Here's how the part is built. I have some questions about the finished solid (model axes, mm). Face numbers are marked on the shaded views. A direction names the side the tool comes from. Round coordinates to 2 decimals unless told otherwise and drop trailing zeros. Order: outer loops, then holes, each group sorted by start corner. A loop starts at its lowest first (then second) coordinate and runs counter-clockwise, first axis right, second up. Notation, with made-up numbers: M 30,69 L 82,69 A21 ccw 82,102 Z; hole C 1.5,19 d10. An arc over 180 degrees is marked long. Write item = value, one per line. Start each with the question number.
Item 1: Please list where these lines run through material, in increasing order: L1, parallel to Y at x = -2.25, z = 0; L2, parallel to Z at x = 0, y = 2.4; L3, parallel to X at y = 2.1, z = -10.5.
Item 2: I want a section at D-D, the plane z = 2. List the corners of the cut face in (x, y) for me, plus the area to 3 significant figures.
Item 3: For the marked faces 1 and 2, which set-ups out of +Z, -Z, +X, -X, +Y, -Y let a thin tool reach every point of the face, with its end or its side?
Item 4: I'm going to push flat-ended pins straight in: P1, Ø6, axis at x = 2, y = 42.5, coming from the -Z side; P2, Ø1, axis at x = -3, z = -3, coming from the +Y side; P3, Ø1.5, axis at x = 3, z = -9, coming from the +Y side. Where does each tip first touch, or does it pass through?
Item 5: I want a section at B-B, the plane z = -10.5. List the corners of the cut face in (x, y) for me.
Item 6: I want a section at A-A, the plane x = 0. State how many separate pieces and enclosed holes the cut face has, plus the area to 3 significant figures.
Item 7: We'd pull the mould along Z, two halves only. Please class the marked faces 3, 4, 5 and 6: pulls with the +Z half, pulls with the -Z half, needs draft (parallel to the pull), parting line crosses it, or undercut.
Autodesk Inventor part; units mm, degrees
ref_plane "YZ Plane" through (0, 0, 0) normal (1, 0, 0) x (0, 1, 0)
ref_plane "XZ Plane" through (0, 0, 0) normal (0, 1, 0) x (-1, 0, 0)
ref_plane "XY Plane" through (0, 0, 0) normal (0, 0, 1) x (1, 0, 0)
sketch "Sketch1" plane through (0, 0, 0) normal (0, 1, 0) x (-1, 0, 0)
  line L0 (7.5, 12.5) -> (-7.5, 12.5)
  line L1 (-7.5, 12.5) -> (-7.5, -12.5)
  line L2 (-7.5, -12.5) -> (7.5, -12.5)
  line L3 (7.5, -12.5) -> (7.5, 12.5)
  line L4 (7.5, 12.5) -> (-7.5, -12.5) construction
  line L5 (-7.5, 12.5) -> (7.5, -12.5) construction
  point P0 (0, 0)
  dimension "d0" = 15
  dimension "d1" = 25
extrude "Extrusion1" add sketch "Sketch1" along normal blind 5
sketch "Sketch2" plane through (0, 5, 0) normal (0, 1, 0) x (1, 0, 0)
  line L0 (-7.5, -12.5) -> (7.5, -12.5)
  line L1 (-7.5, 12.5) -> (-7.5, -12.5)
  line L2 (7.5, 7.5) -> (-7.5, 7.5)
  line L3 (-7.5, 7.5) -> (-7.5, -7.5)
  line L4 (-7.5, -7.5) -> (7.5, -7.5)
  line L5 (7.5, -7.5) -> (7.5, 7.5)
  line L6 (7.5, 7.5) -> (-7.5, -7.5) construction
  line L7 (-7.5, 7.5) -> (7.5, -7.5) construction
  point P0 (0, 0)
  dimension "d5" = 15
extrude "Extrusion2" add sketch "Sketch2" along normal blind 50
sketch "Sketch3" plane through (7.5, 0, 12.5) normal (1, 0, 0) x (0, 0, -1)
  circle A0 centre (12.5, 47.5) radius 5.5
  point P0 (12.5, 0)
  point P1 (14.5, 47.5)
  dimension "d9" = 11
extrude "Extrusion3" cut sketch "Sketch3" against normal blind 13
fillet "Fillet1" radius 7.5 2 edges at (0, 55, -7.5) (0, 55, 7.5)
sketch "Sketch5" plane through (0, 5, 0) normal (0, 1, 0) x (1, 0, 0)
  line L0 (7.5, -7.5) -> (-7.5, -7.5)
  line L1 (-7.5, -12.5) -> (7.5, -12.5)
  line L2 (-7.5, 7.5) -> (7.5, 7.5)
  line L3 (7.5, 12.5) -> (-7.5, 12.5)
  point P0 (0, 0)
  point P1 (0, -10.5)
  point P2 (0, 10.5)
hole "Hole2" at (0, 5, 10.5) at (0, 5, -10.5) direction (0, -1, 0) diameter 3.5 end through all
sketch "Sketch6" plane through (0, 5, 0) normal (0, 1, 0) x (1, 0, 0)
  point P0 (0, 0)
sketch "Sketch7" plane through (0, 5, 0) normal (0, 1, 0) x (1, 0, 0)
  line L0 (7.5, -7.5) -> (-7.5, -7.5)
  line L1 (-7.5, -12.5) -> (7.5, -12.5)
  line L2 (-7.5, -7.5) -> (7.5, -7.5)
  line L3 (7.5, -7.5) -> (7.5, -12.5)
  line L4 (7.5, -12.5) -> (-7.5, -12.5)
  line L5 (-7.5, -12.5) -> (-7.5, -7.5)
  line L6 (-7.5, -12.5) -> (7.5, -12.5)
  line L7 (7.5, -12.5) -> (7.5, -8.5)
  line L8 (7.5, -8.5) -> (-7.5, -8.5)
  line L9 (-7.5, -8.5) -> (-7.5, -12.5)
  point P0 (0, 0)
  point P1 (-7.5, -8.5)
  dimension "d33" = 4
extrude "Extrusion5" cut sketch "Sketch7" against normal through all contours L3 L1 L5 L8
properties part number "Holder_slim_1_fod_højre"
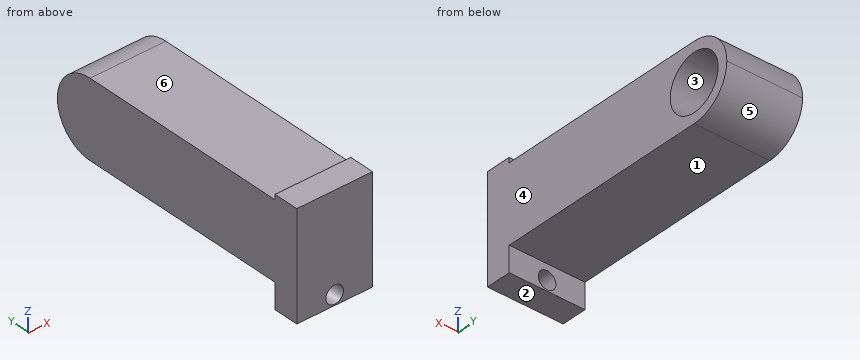
Filled in:
q1.L1 = 0 to 42, 53 to 55
q1.L2 = -12.5 to -12.25, -8.75 to 8.5
q1.L3 = -7.5 to -1.75, 1.75 to 7.5
q2.outline = M -7.5,0 L 7.5,0 L 7.5,42.38 L -5.5,42.38 L -5.5,52.62 L 7.5,52.62 L 7.5,54.73 L -7.5,54.73 Z
q2.area = 688 mm^2
q3.face_1 = -Z, +X, -X, +Y
q3.face_2 = -Z, +X, -X, +Y, -Y
q4.P1 = -7.5
q4.P2 = 54.57
q4.P3 = 5
q5.outline = M -7.5,0 L -1.75,0 L -1.75,5 L -7.5,5 Z; M 1.75,0 L 7.5,0 L 7.5,5 L 1.75,5 Z
q6.separate_pieces = 2
q6.enclosed_holes = 1
q6.area = 718 mm^2
q7.face_3 = undercut
q7.face_4 = needs draft
q7.face_5 = pulls with the -Z half
q7.face_6 = pulls with the +Z half
